Geometry check sheet. Reference: the model listing, model coordinates, mm. Face numbers are marked on the shaded views. A direction names the side the tool comes from. Round coordinates to 2 decimals unless told otherwise and drop trailing zeros. Write each loop counter-clockwise with the first axis right and the second up, starting at its lowest first coordinate (ties: lowest second). Pieces come first, ordered by that corner, then holes. Notation, with made-up numbers: (-12, -7) -> (37, -7) arc R14 ccw to (37, 0) -> close; hole circle Ø2 at (23.5, 81.25). An arc over 180 degrees is marked (long way). Use a Markdown table: item, result.
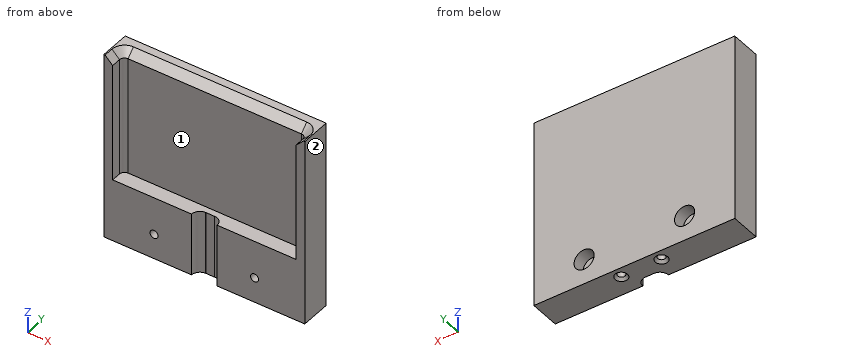
```python
from build123d import *

# Parameters (mm, degrees)
F0_R     = 1.475
F1_DEPTH = 25
F2_R     = 1.6
F3_DEPTH = 30
F2_R_2   = 4
F4_DEPTH = 5
F5_R     = 1.475
F6_DEPTH = 50
F7_SIZE  = 3
F8_DEPTH = 20
F9_SIZE  = 1


with BuildPart() as f1:
    # F0 (on Top) → F1 (new body)
    with BuildSketch(Plane.XY):
        with BuildLine():
            ThreePointArc((-5.1, 0), (-4.141202, 2.3462), (-1.81364, 3.349395))
            ThreePointArc((-1.81364, 3.349395), (-1.750568, 3.35), (-1.687497, 3.349417))
            Line((-1.687497, 3.349417), (1.749432, 3.35))
            ThreePointArc((1.749432, 3.35), (4.118607, 2.369009), (5.1, 0))
            Line((5.1, 0), (40, 0))
            Line((40, 0), (40, 12))
            Line((40, 12), (-40, 12))
            Line((-40, 12), (-40, 0))
            Line((-40, 0), (-5.1, 0))
        make_face()
        with Locations((-8, 8)):
            Circle(F0_R, mode=Mode.SUBTRACT)
        with Locations((8, 8)):
            Circle(F0_R, mode=Mode.SUBTRACT)
    extrude(amount=F1_DEPTH)

    # F2 (on face) → F3 (cut)
    with BuildSketch(Plane(origin=(0, 12, 0), x_dir=(-1, 0, 0), z_dir=(0, 1, 0))):
        with Locations((-20, 10)):
            Circle(F2_R)
        with Locations((20, 10)):
            Circle(F2_R)
    extrude(amount=-F3_DEPTH, mode=Mode.SUBTRACT)

    # F2 (on face) → F4 (cut)
    with BuildSketch(Plane(origin=(0, 12, 0), x_dir=(-1, 0, 0), z_dir=(0, 1, 0))):
        with Locations((-20, 10)):
            Circle(F2_R_2)
        with Locations((-20, 10)):
            Circle(F2_R, mode=Mode.SUBTRACT)
        with Locations((20, 10)):
            Circle(F2_R_2)
        with Locations((20, 10)):
            Circle(F2_R, mode=Mode.SUBTRACT)
    extrude(amount=-F4_DEPTH, mode=Mode.SUBTRACT)

    # F5 (on face) → F6 (join)
    with BuildSketch(Plane.XY.offset(25)):
        with BuildLine():
            Line((40, 12), (-40, 12))
            Line((-40, 12), (-40, 0))
            Line((-40, 0), (-36.5, 0))
            Line((-36.5, 0), (-36.5, 3.849708))
            ThreePointArc((-36.5, 3.849708), (-35.914214, 5.263922), (-34.5, 5.849708))
            Line((-34.5, 5.849708), (34.5, 5.849708))
            ThreePointArc((34.5, 5.849708), (35.914214, 5.263922), (36.5, 3.849708))
            Line((36.5, 3.849708), (36.5, 0))
            Line((36.5, 0), (40, 0))
            Line((40, 0), (40, 12))
        make_face()
        with Locations((-8, 8)):
            Circle(F5_R, mode=Mode.SUBTRACT)
        with Locations((8, 8)):
            Circle(F5_R, mode=Mode.SUBTRACT)
        with Locations((-8, 8)):
            Circle(F5_R)
        with Locations((8, 8)):
            Circle(F5_R)
    extrude(amount=F6_DEPTH)

    # F7
    f7_edges = [f1.edges().sort_by_distance(p)[0] for p in [
        (0, 5.849708, 75),
    ]]
    chamfer(f7_edges, length=F7_SIZE)

    # F0 (on Top) → F8 (cut)
    with BuildSketch(Plane.XY):
        with Locations((-8, 8)):
            Circle(F0_R)
        with Locations((8, 8)):
            Circle(F0_R)
    extrude(amount=F8_DEPTH, mode=Mode.SUBTRACT)

    # F9
    f9_edges = [f1.edges().sort_by_distance(p)[0] for p in [
        (-9.475, 8, 0),
        (6.525, 8, 0),
    ]]
    chamfer(f9_edges, length=F9_SIZE)


solid = f1.part
```
(1) Thickness scan on line 1 (Z direction, x = -20, y = 10.15); line 2 (Z direction, x = 20, y = 1.5); line 3 (Y direction, x = 8, z = 11) (3 decimals). Record the ranges inside material, lowest first.
A:
| item | result |
|---|---|
| line 1 | z = 0 to 6, 14 to 75 |
| line 2 | z = 0 to 8.4, 11.6 to 25 |
| line 3 | y = 0 to 6.525, 9.475 to 12 |
(2) Section check B-B on x = -20. Record the cut outline in (y, z), plus the area to 3 significant figures.
A:
| item | result |
|---|---|
| outline | (0, 0) -> (12, 0) -> (12, 6) -> (7, 6) -> (7, 8.4) -> (0, 8.4) -> close; (0, 11.6) -> (7, 11.6) -> (7, 14) -> (12, 14) -> (12, 75) -> (8.85, 75) -> (5.85, 72) -> (5.85, 25) -> (0, 25) -> close |
| area | 541 mm2 |
(3) Section check A-A on z = 10. State how many separate pieces and enclosed holes the cut face has, plus the area to 3 significant figures.
A:
| item | result |
|---|---|
| separate pieces | 3 |
| enclosed holes | 2 |
| area | 792 mm2 |
(4) Gauge pin test, flat ends, axial feed: pin 1 Ø14 at (x, z) = (-17, 56.5) entering from -Y; pin 2 Ø1.5 at (x, y) = (1, 6) entering from +Z; pin 3 Ø1.9 at (x, z) = (20, 10) entering from +Y; pin 4 Ø2.5 at (x, y) = (8.5, 7.5) entering from -Z. Record the tip position at first contact, or that the pin passes through.
A:
| item | result |
|---|---|
| pin 1 | stops at y = 5.85 |
| pin 2 | stops at z = 72.9 |
| pin 3 | passes through |
| pin 4 | stops at z = 0.52 |
(5) Section check C-C on y = 1.5. Record the cut outline in (x, z), plus the area to 3 significant figures.
A:
| item | result |
|---|---|
| outline | (-40, 0) -> (-4.75, 0) -> (-4.75, 25) -> (-36.5, 25) -> (-36.5, 72) -> (-39.5, 75) -> (-40, 75) -> close; (4.75, 0) -> (40, 0) -> (40, 75) -> (39.5, 75) -> (36.5, 72) -> (36.5, 25) -> (4.75, 25) -> close; hole circle Ø3.2 at (-20, 10); hole circle Ø3.2 at (20, 10) |
| area | 2,090 mm2 |
(6) Access from +Z, -Z, +X, -X, +Y, -Y to the whole of each face (thin tool, end or side, straight path). Record for the marked faces 1 and 2.
A:
| item | result |
|---|---|
| face 1 | +Z, -Y |
| face 2 | +Z, -Z, +X, +Y, -Y |
